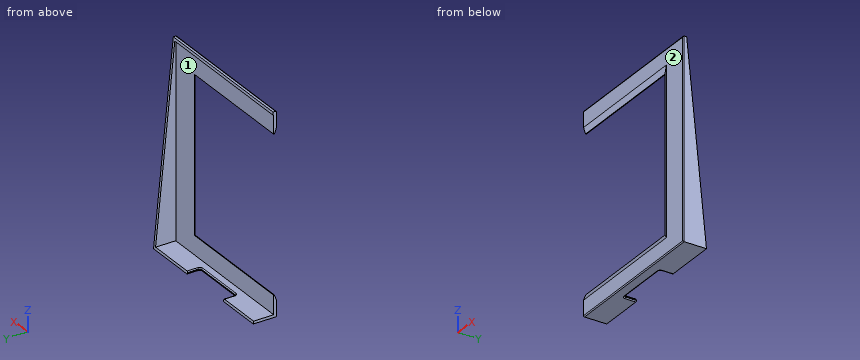
from build123d import *
from OCP.BRepFilletAPI import BRepFilletAPI_MakeChamfer

# Parameters (mm, degrees)
CROQUIS1_W                 = 220.407444928
CROQUIS1_H                 = 139.358729484
CROQUIS1_W_2               = 180
CROQUIS1_H_2               = 113.81
SALIENTE_EXTRUIR1_DEPTH    = 2
EXTRUIR_L_MINA3_DEPTH      = 16.5
EXTRUIR_L_MINA3_DEPTH_BACK = 2
CROQUIS2_W                 = 226.407444928
CROQUIS2_H                 = 145.358729484
CROQUIS2_W_2               = 220.407444928
CROQUIS2_H_2               = 139.358729484
CROQUIS6_W                 = 222.447038553
CROQUIS6_H                 = 141.398323109
CORTAR_EXTRUIR2_DEPTH      = 16.5
CORTAR_EXTRUIR3_REACH      = 240.505
CORTAR_EXTRUIR4_DEPTH      = 1.960406375
REDONDEO2_R                = 0.7
CHAFL_N1_SIZE              = 1.5
CHAFL_N1_SIZE2             = 4.121216129
REDONDEO3_R                = 0.7


with BuildPart() as part:
    # Croquis1 → Saliente-Extruir1 (new body)
    with BuildSketch(Plane(origin=(0, 0, 0), x_dir=(1, 0, 0), z_dir=(0, 1, 0))):
        Rectangle(CROQUIS1_W, CROQUIS1_H)
        Rectangle(CROQUIS1_W_2, CROQUIS1_H_2, mode=Mode.SUBTRACT)
    extrude(amount=SALIENTE_EXTRUIR1_DEPTH)

    # Croquis2 → Extruir-Lámina3 (add, two sides: drawn at the far end of the back side and taken through both)
    with BuildSketch(Plane(origin=(0, 2, 0), x_dir=(1, 0, 0), z_dir=(0, 1, 0)).offset(-EXTRUIR_L_MINA3_DEPTH_BACK)):
        Rectangle(CROQUIS2_W, CROQUIS2_H)
        Rectangle(CROQUIS2_W_2, CROQUIS2_H_2, mode=Mode.SUBTRACT)
    extrude(amount=EXTRUIR_L_MINA3_DEPTH + EXTRUIR_L_MINA3_DEPTH_BACK)

    # Croquis6 → Cortar-Extruir2 (cut)
    with BuildSketch(Plane(origin=(0, 18.5, 0), x_dir=(1, 0, 0), z_dir=(0, 1, 0))):
        with Locations((-0.019796812, 0.019796812)):
            Rectangle(CROQUIS6_W, CROQUIS6_H)
    extrude(amount=-CORTAR_EXTRUIR2_DEPTH, mode=Mode.SUBTRACT)

    # Cortar-Extruir3: up to this face of the body (flat: up to its plane)
    cortar_extruir3_end = Plane(part.part.faces().sort_by_distance((113.203722464, 9.25, 0))[0])
    # Croquis7 → Cortar-Extruir3 (cut, up to the picked face)
    with BuildSketch(Plane.ZY.offset(113.203722464), mode=Mode.PRIVATE) as cortar_extruir3_sk1:
        Polygon((-72.679364742, 18.5), (-72.679364742, 17.034353119), (72.679364742, 2.5), (72.679364742, 18.5), align=None)
    cortar_extruir3_tool1 = split(extrude(cortar_extruir3_sk1.sketch, amount=-CORTAR_EXTRUIR3_REACH, mode=Mode.PRIVATE), bisect_by=cortar_extruir3_end, keep=Keep.BOTH, mode=Mode.PRIVATE)
    add(cortar_extruir3_tool1.solids().sort_by(Axis((-113.203722, 13.12567, 20.160481), (1, 0, 0)))[0], mode=Mode.SUBTRACT)

    # Croquis8 → Cortar-Extruir4 (cut)
    with BuildSketch(Plane(origin=(0, 0, -72.679364742), x_dir=(-1, 0, 0), z_dir=(0, 0, -1))):
        with BuildLine():
            Line((-33.703722464, 17.034353119), (-74.703722464, 17.034353119))
            Line((-74.703722464, 17.034353119), (-74.703722464, 9.034353119))
            ThreePointArc((-74.703722464, 9.034353119), (-74.264382636, 7.973692947), (-73.203722464, 7.534353119))
            Line((-73.203722464, 7.534353119), (-35.203722464, 7.534353119))
            ThreePointArc((-35.203722464, 7.534353119), (-34.143062292, 7.973692947), (-33.703722464, 9.034353119))
            Line((-33.703722464, 9.034353119), (-33.703722464, 17.034353119))
        make_face()
    extrude(amount=-CORTAR_EXTRUIR4_DEPTH, mode=Mode.SUBTRACT)

    # Redondeo2
    redondeo2_edges = [part.edges().sort_by_distance(p)[0] for p in [
        (33.703722464, 12.936343049, -70.718958367),
        (34.143062292, 7.973692947, -70.718958367),
        (54.203722464, 7.534353119, -70.718958367),
        (74.264382636, 7.973692947, -70.718958367),
        (74.703722464, 12.936343049, -70.718958367),
        (74.703722464, 13.034353119, -72.679364742),
        (74.264382636, 7.973692947, -72.679364742),
        (54.203722464, 7.534353119, -72.679364742),
        (34.143062292, 7.973692947, -72.679364742),
        (33.703722464, 13.034353119, -72.679364742),
    ]]
    fillet(redondeo2_edges, radius=REDONDEO2_R)

    # Chaflán1: one chamfer whose edges measure the first distance from different faces: ONE call of the kernel's chamfer builder (chamfer() names one face for all edges)
    chafl_n1_edges_1 = [part.edges().sort_by_distance(p)[0] for p in [
        (90, 0, 0),
    ]]
    chafl_n1_side_1 = [part.faces().sort_by_distance(p)[0] for p in [
        (90, 1, 0),
    ]]
    chafl_n1_edges_2 = [part.edges().sort_by_distance(p)[0] for p in [
        (0, 0, -56.905),
    ]]
    chafl_n1_side_2 = [part.faces().sort_by_distance(p)[0] for p in [
        (0, 1, -56.905),
    ]]
    chafl_n1_edges_3 = [part.edges().sort_by_distance(p)[0] for p in [
        (-90, 0, 0),
    ]]
    chafl_n1_side_3 = [part.faces().sort_by_distance(p)[0] for p in [
        (-90, 1, 0),
    ]]
    chafl_n1_edges_4 = [part.edges().sort_by_distance(p)[0] for p in [
        (0, 0, 56.905),
    ]]
    chafl_n1_side_4 = [part.faces().sort_by_distance(p)[0] for p in [
        (0, 1, 56.905),
    ]]
    chafl_n1 = BRepFilletAPI_MakeChamfer(part.part.solid().wrapped)
    for e in chafl_n1_edges_1:
        chafl_n1.Add(CHAFL_N1_SIZE, CHAFL_N1_SIZE2, e.wrapped, chafl_n1_side_1[0].wrapped)  # the first distance lies on this face
    for e in chafl_n1_edges_2:
        chafl_n1.Add(CHAFL_N1_SIZE, CHAFL_N1_SIZE2, e.wrapped, chafl_n1_side_2[0].wrapped)  # the first distance lies on this face
    for e in chafl_n1_edges_3:
        chafl_n1.Add(CHAFL_N1_SIZE, CHAFL_N1_SIZE2, e.wrapped, chafl_n1_side_3[0].wrapped)  # the first distance lies on this face
    for e in chafl_n1_edges_4:
        chafl_n1.Add(CHAFL_N1_SIZE, CHAFL_N1_SIZE2, e.wrapped, chafl_n1_side_4[0].wrapped)  # the first distance lies on this face
    add(Compound.cast(chafl_n1.Shape()), mode=Mode.REPLACE)

    # Redondeo3
    redondeo3_edges = [part.edges().sort_by_distance(p)[0] for p in [
        (-113.203722464, 0, 0),
        (0, 0, -72.679364742),
        (113.203722464, 0, 0),
        (0, 0, 72.679364742),
    ]]
    fillet(redondeo3_edges, radius=REDONDEO3_R)

    # Partir2
    split(bisect_by=Plane(origin=(0, 0, 0), x_dir=(0, 0, 1), z_dir=(1, 0, 0)), keep=Keep.TOP)


solid = part.part
Geometry check sheet. Reference: the model listing, model coordinates, mm. Face numbers are marked on the shaded views. A direction names the side the tool comes from. Round coordinates to 2 decimals unless told otherwise and drop trailing zeros. Write each loop counter-clockwise with the first axis right and the second up, starting at its lowest first coordinate (ties: lowest second). Pieces come first, ordered by that corner, then holes.
Item 1: Section check B-B (y = 11.5). Record the boundary of the cut face in (x, z), plus the area to 3 significant figures.
Determined:
outline: (0, -72.68) - (33, -72.68) arc R0.7 ccw to (33.7, -71.98) - (33.7, -71.42) arc R0.7 ccw to (33, -70.72) - (0, -70.72) - close; (74.7, -71.98) arc R0.7 ccw to (75.4, -72.68) - (113.2, -72.68) - (113.2, -17.33) - (111.2, -17.33) - (111.2, -70.72) - (75.4, -70.72) arc R0.7 ccw to (74.7, -71.42) - close
area: 248 mm2
Item 2: Section check D-D (z = -40.5). Record the boundary of the cut face in (x, y), plus the area to 3 significant figures.
Determined:
outline: (90, 1.5) - (94.12, 0) - (112.5, 0) arc R0.7 ccw to (113.2, 0.7) - (113.2, 13.82) - (111.2, 13.82) - (111.2, 2) - (90, 2) - close
area: 66.8 mm2
Item 3: Go/stop test with flat-tipped pins: pin 1 Ø0.6 at (y, z) = (1.5, 9) entering from -X; pin 2 Ø12 at (x, z) = (86, -38.5) entering from -Y; pin 3 Ø6 at (y, z) = (9.5, -0.5) entering from -X. Record where each tip stops, or that it passes through.
Determined:
pin 1: stops at x = 90
pin 2: stops at y = 0.77
pin 3: stops at x = 111.2
Item 4: Section check A-A (x = 82). Record the boundary of the cut face in (y, z) (3 decimals).
Determined:
outline: (0, -71.979) arc R0.7 ccw to (0.7, -72.679) - (17.034, -72.679) - (16.838, -70.719) - (2, -70.719) - (2, -56.905) - (1.5, -56.905) - (0, -61.026) - close; (0, 61.026) - (1.5, 56.905) - (2, 56.905) - (2, 70.679) - (2.7, 70.679) - (2.5, 72.679) - (0.7, 72.679) arc R0.7 ccw to (0, 71.979) - close
Item 5: Material ranges on line 1 along X through (y, z) = (9, -12.5); line 2 along Z through (x, y) = (60.5, 6.5); line 3 along Y through (x, z) = (101.5, 51), recorded low to high.
Determined:
line 1: x = 111.2 to 113.2
line 2: z = -72.68 to -70.72
line 3: y = 0 to 2
Item 6: Access from +Z, -Z, +X, -X, +Y, -Y to the whole of each face (thin tool, end or side, straight path). Record for the marked faces 1 and 2.
Determined:
face 1: -X, +Y
face 2: +Z, -Z, +X, -X, -Y
Item 7: Section check C-C (z = 49). Record the boundary of the cut face in (x, y), plus the area to 3 significant figures.
Determined:
outline: (90, 1.5) - (94.12, 0) - (112.5, 0) arc R0.7 ccw to (113.2, 0.7) - (113.2, 4.87) - (111.2, 4.87) - (111.2, 2) - (90, 2) - close
area: 48.9 mm2
